from build123d import *

# Parameters (mm, degrees)
F0_R     = 3.175
F1_DEPTH = 228.6
F2_W     = 50.8
F2_H     = 3.2004
F3_DEPTH = 12.7


with BuildPart() as f1:
    # F0 (on Top) → F1 (new body, symmetric)
    with BuildSketch(Plane.XY):
        Circle(F0_R)
    extrude(amount=F1_DEPTH, both=True)

    # F2 (on Front) → F3 (cut, symmetric)
    with BuildSketch(Plane.XZ):
        with Locations((-23.8125, -177.8)):
            Rectangle(F2_W, F2_H)
        with Locations((-23.8125, -47.5996)):
            Rectangle(F2_W, F2_H)
        with Locations((-23.8125, 82.6008)):
            Rectangle(F2_W, F2_H)
    extrude(amount=F3_DEPTH, both=True, mode=Mode.SUBTRACT)


solid = f1.part
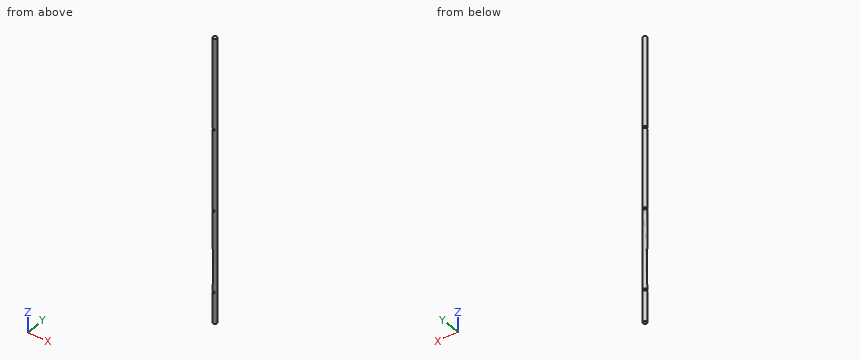
Build history of the part. All positions in model axes, mm. Give positions to 0.01 mm unless a question says otherwise; leave off trailing zeros. Write each loop counter-clockwise with the first axis right and the second up, starting at its lowest first coordinate (ties: lowest second). Pieces come first, ordered by that corner, then holes. Notation, with made-up numbers: (71, 1.25) - (83, 1.25) arc R27 ccw to (83, 39.25) - close; hole circle Ø11 at (-17, 9). An arc over 180 degrees is marked (long way). Use one line per item in the form item = value. Start each with the question number.
1. Band-saw the part on A-A on x = 0. Write the cut outline in (y, z) (3 decimals).
2. Drop flat-ended pins along their axis: pin 1 Ø1.5 at (y, z) = (1, 159) entering from -X; pin 2 Ø1.6 at (y, z) = (-1, -48.5) entering from -X; pin 3 Ø1 at (y, z) = (-1, 83) entering from -X. Give the stop position or say it passes through.
3. Band-saw the part on C-C on z = 156. Write the cut outline in (x, y) (3 decimals), plus the area to 3 significant figures.
4. Band-saw the part on B-B on y = 0. Write the cut outline in (x, z) (1 decimal).
5. Probe line 1 (Z direction, x = 0, y = 2.25); line 2 (X direction, y = 0.5, z = -24). List the from-to ranges inside material, lowest first. Write a range as [from, to].
Conclusion:
q1.outline = (-3.175, -228.6) - (3.175, -228.6) - (3.175, -179.4) - (-3.175, -179.4) - close; (-3.175, -176.2) - (3.175, -176.2) - (3.175, -49.2) - (-3.175, -49.2) - close; (-3.175, -45.999) - (3.175, -45.999) - (3.175, 81.001) - (-3.175, 81.001) - close; (-3.175, 84.201) - (3.175, 84.201) - (3.175, 228.6) - (-3.175, 228.6) - close
q2.pin_1 = -3.17
q2.pin_2 = -3.12
q2.pin_3 = 1.59
q3.outline = circle Ø6.35 at (0, 0)
q3.area = 31.7 mm²
q4.outline = (-3.2, -228.6) - (3.2, -228.6) - (3.2, 228.6) - (-3.2, 228.6) - (-3.2, 84.2) - (1.6, 84.2) - (1.6, 81) - (-3.2, 81) - (-3.2, -46) - (1.6, -46) - (1.6, -49.2) - (-3.2, -49.2) - (-3.2, -176.2) - (1.6, -176.2) - (1.6, -179.4) - (-3.2, -179.4) - close
q5.line_1 = [-228.6, -179.4], [-176.2, -49.2], [-46, 81], [84.2, 228.6]
q5.line_2 = [-3.14, 3.14]
